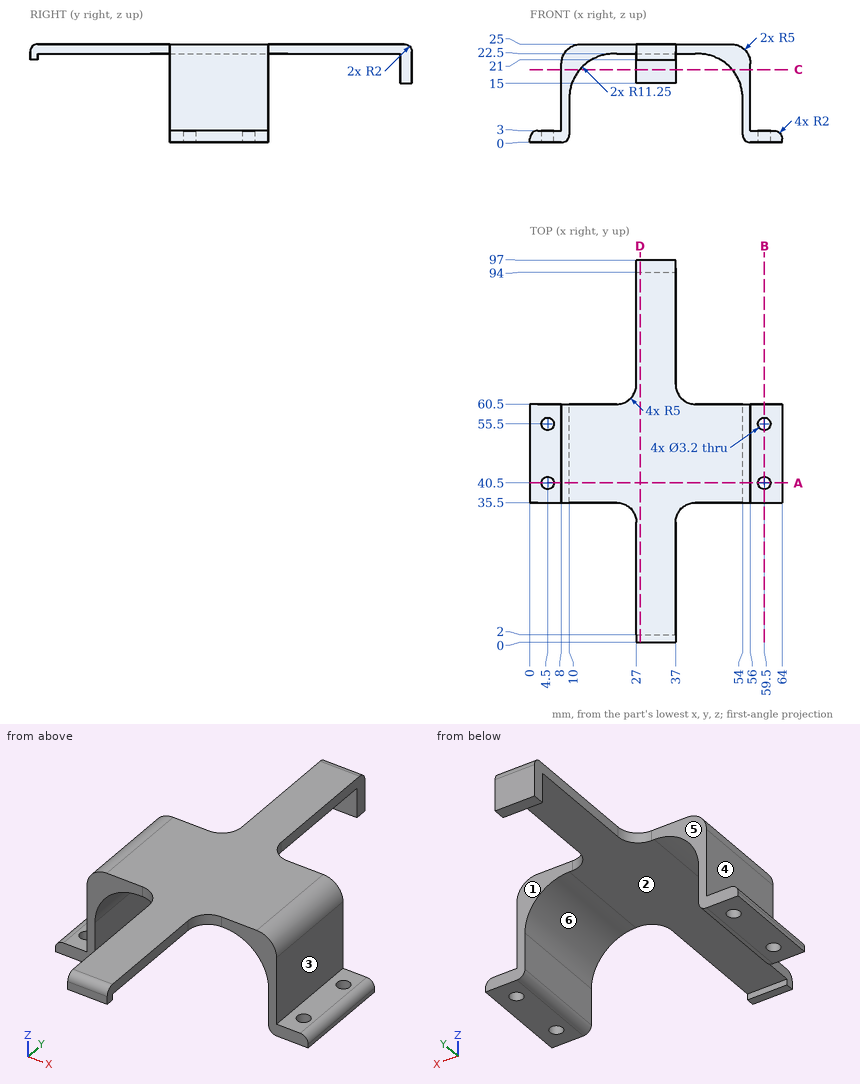
Design review of the part shown in the three views and the two pictorial views. Dimensions are in mm from the part's minimum x, y and z. A direction names the side the tool comes from. Round coordinates to 2 decimals unless told otherwise and drop trailing zeros. Write each loop counter-clockwise with the first axis right and the second up, starting at its lowest first coordinate (ties: lowest second). Pieces come first, ordered by that corner, then holes.
Item 1: For probe 1 along Y at (x, z) = (4.5, 1.6); probe 2 along X at (y, z) = (40.5, 2.35); probe 3 along X at (y, z) = (40.5, 1), list the stretches that pass through material, from the lowest coordinate up.
Item 2: For the marked faces 1, 2 and 3, list the 3-axis set-ups (+Z, -Z, +X, -X, +Y, -Y) from which the entire face can be reached by the end or side of a thin tool; tool diameter is ignored.
Item 3: We need section C-C on z = 18.5. Write out the cut boundary in (x, y).
Item 4: Clearance check with flat-ended pins moving along their axes: pin 1 Ø2 at (x, z) = (32.5, 19.5) entering from -Y; pin 2 Ø3 at (y, z) = (81, 21.5) entering from +X; pin 3 Ø5 at (x, y) = (4.5, 40.5) entering from +Z. State where each tip first meets the part, or that it passes through.
Item 5: We need section B-B on x = 59.5. Write out the cut boundary in (y, z).
Item 6: We need section D-D on x = 28. Write out the cut boundary in (y, z).
Item 7: The part is to be moulded in two halves that separate along X. For the marked faces 4, 5 and 6, say which applies: +X half, -X half, draft (parallel to the pull), parting line (faces both ways), or undercut.
Item 8: We need section A-A on y = 40.5. Write out the cut boundary in (x, z), and give its area (3 significant figures).
Returned:
1. probe 1: y = 35.5 to 38.9, 42.1 to 53.9, 57.1 to 60.5
1. probe 2: x = 0.52 to 2.9, 6.1 to 10, 54 to 57.9, 61.1 to 63.48
1. probe 3: x = 0 to 2.9, 6.1 to 9.73, 54.27 to 57.9, 61.1 to 64
2. face 1: +Z, -Z, +X, +Y
2. face 2: -Z
2. face 3: +Z, +X, +Y, -Y
3. outline: (8, 35.5) - (12.65, 35.5) - (12.65, 60.5) - (8, 60.5) - close; (27, 94) - (37, 94) - (37, 97) - (27, 97) - close; (51.35, 35.5) - (56, 35.5) - (56, 60.5) - (51.35, 60.5) - close
4. pin 1: stops at y = 94
4. pin 2: stops at x = 37
4. pin 3: stops at z = 3
5. outline: (35.5, 0) - (38.9, 0) - (38.9, 3) - (35.5, 3) - close; (42.1, 0) - (53.9, 0) - (53.9, 3) - (42.1, 3) - close; (57.1, 0) - (60.5, 0) - (60.5, 3) - (57.1, 3) - close
6. outline: (0, 21) - (2, 21) - (2, 22.5) - (94, 22.5) - (94, 15) - (97, 15) - (97, 23) arc R2 ccw to (95, 25) - (2, 25) arc R2 ccw to (0, 23) - close
7. face 4: -X half
7. face 5: draft
7. face 6: undercut
8. outline: (0, 0) - (2.9, 0) - (2.9, 3) - (2, 3) arc R2 ccw to (0, 1) - close; (6.1, 0) - (8, 0) arc R2 ccw to (10, 2) - (10, 11.25) arc R11.25 cw to (21.25, 22.5) - (42.75, 22.5) arc R11.25 cw to (54, 11.25) - (54, 2) arc R2 ccw to (56, 0) - (57.9, 0) - (57.9, 3) - (56, 3) - (56, 20) arc R5 ccw to (51, 25) - (13, 25) arc R5 ccw to (8, 20) - (8, 3) - (6.1, 3) - close; (61.1, 0) - (64, 0) - (64, 1) arc R2 ccw to (62, 3) - (61.1, 3) - close
8. area: 279 mm2
